Verification items for this drawing (mm, ordinates from the low corner). A direction names the side the tool comes from. Give positions to 0.01 mm unless a question says otherwise; leave off trailing zeros. Loops run counter-clockwise (first coordinate to the right, second up) from the corner with the lowest first, then second, coordinate; pieces in that order, holes last. Notation, with made-up numbers: (37.5, 85.5) -> (61.5, 85.5) arc R20 cw to (61.5, 123.5) -> close; hole circle Ø4 at (77, 51.5). An arc over 180 degrees is marked (long way). Write each question's results on one line, items separated by ' | '. Start each with the question number.
1) Depth check by flat-ended pin: pin 1 (1 mm diameter, centred on y = 14, z = 4, fed in from +X); pin 2 (1.5 mm diameter, centred on x = 3.5, z = 9, fed in from +Y). Enter the tip coordinate at first touch or a pass-through.
2) Sectioned sample at D-D on z = 3. Record the cut outline in (x, y).
3) Scan lines: line 1 (Y direction, x = 4.75, z = 3); line 2 (Y direction, x = 3.75, z = 3); line 3 (Y direction, x = 4.5, z = 14.75). Record each from-to range of solid material in increasing order. Write a range as from..to.
4) Sectioned sample at A-A on x = 3.75. Record the cut outline in (y, z).
5) Sectioned sample at B-B on y = 7. Record the cut outline in (x, z), then the cut area to 3 significant figures.
6) Draft check along Y on the marked faces 3, 4, 5 and 6. Enter one of: pulls with the +Y half, pulls with the -Y half, needs draft (parallel to the pull), parting line crosses it, or undercut.
7) Set-up check for the marked faces 1 and 2: record each of +Z, -Z, +X, -X, +Y, -Y from which the full face is reachable in a straight line by a thin tool's end or side.
8) Sectioned sample at C-C on x = 1.25. Record the cut outline in (y, z), then the cut area to 3 significant figures.
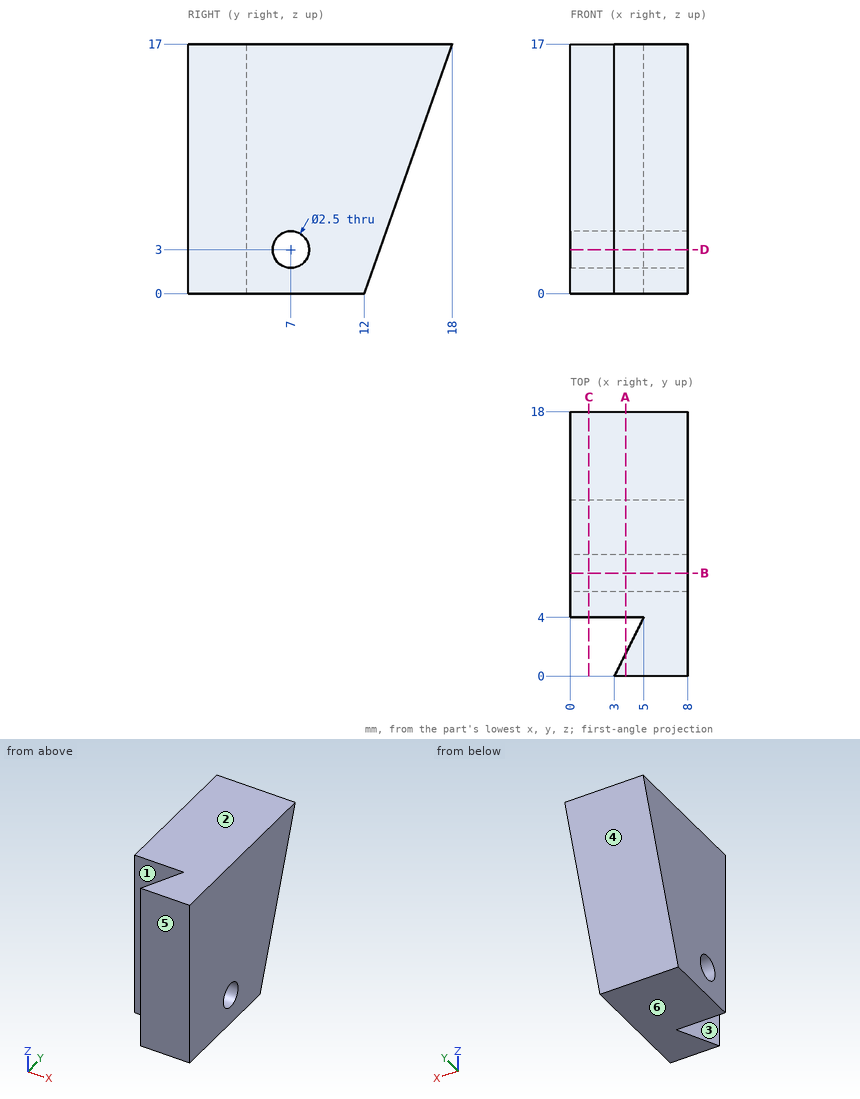
Result:
1) pin 1: through | pin 2: y = 15.44
2) outline: (0, 4) -> (5, 4) -> (3, 0) -> (8, 0) -> (8, 5.75) -> (0, 5.75) -> close; (0, 8.25) -> (8, 8.25) -> (8, 13.06) -> (0, 13.06) -> close
3) line 1: 0..3.5, 4..5.75, 8.25..13.06 | line 2: 0..1.5, 4..5.75, 8.25..13.06 | line 3: 0..3, 4..17.21
4) outline: (0, 0) -> (1.5, 0) -> (1.5, 17) -> (0, 17) -> close; (4, 0) -> (12, 0) -> (18, 17) -> (4, 17) -> close; hole circle Ø2.5 at (7, 3)
5) outline: (0, 0) -> (8, 0) -> (8, 1.75) -> (0, 1.75) -> close; (0, 4.25) -> (8, 4.25) -> (8, 17) -> (0, 17) -> close | area: 116 mm^2
6) face 3: undercut | face 4: pulls with the +Y half | face 5: pulls with the -Y half | face 6: needs draft
7) face 1: +Z, -Z, -X | face 2: +Z, +X, -X, +Y, -Y
8) outline: (4, 0) -> (12, 0) -> (18, 17) -> (4, 17) -> close; hole circle Ø2.5 at (7, 3) | area: 182 mm^2
